Check sheet for the modelled part. Datum: model origin and axes. Units: mm. Face numbers are marked on the shaded views. A direction names the side the tool comes from. Coordinates: 2 decimals unless noted, no trailing zeros. Write each loop counter-clockwise with the first axis right and the second up, starting at its lowest first coordinate (ties: lowest second). Pieces come first, ordered by that corner, then holes. Notation, with made-up numbers: (19.25, -37.75) - (75.25, -37.75) arc R11 ccw to (75.25, -26.75) - close; hole circle Ø10 at (4, 42). An arc over 180 degrees is marked (long way). Answer as CSV lines item,"result". Start each with the question number.
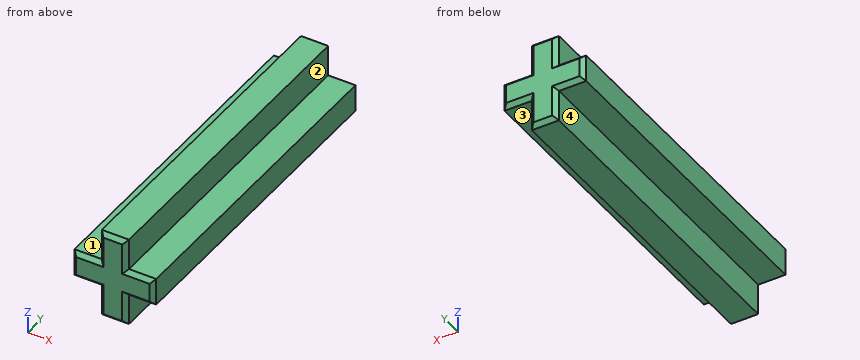
from build123d import *

# Parameters (mm, degrees)
SKETCH1_W           = 1.635
SKETCH1_H           = 1.63
SKETCH1_W_2         = 1.63
SKETCH1_H_2         = 1.87
BOSS_EXTRUDE1_DEPTH = 20
CHAMFER1_SIZE       = 0.25
CHAMFER2_SIZE       = 0.25


with BuildPart() as part:
    # Sketch1 → Boss-Extrude1 (new body)
    with BuildSketch(Plane(origin=(0, 0, 0), x_dir=(1, 0, 0), z_dir=(0, 1, 0))):
        with Locations((-0.8175, 2.685)):
            Rectangle(SKETCH1_W, SKETCH1_H)
        with Locations((0.815, 2.685)):
            Rectangle(SKETCH1_W_2, SKETCH1_H)
        with Locations((0.815, 4.435)):
            Rectangle(SKETCH1_W_2, SKETCH1_H_2)
        with Locations((2.4475, 2.685)):
            Rectangle(SKETCH1_W, SKETCH1_H)
        with Locations((0.815, 0.935)):
            Rectangle(SKETCH1_W_2, SKETCH1_H_2)
    extrude(amount=BOSS_EXTRUDE1_DEPTH)

    # Chamfer1
    chamfer1_edges = [part.edges().sort_by_distance(p)[0] for p in [
        (-0.8175, 20, -1.87),
        (0, 20, -0.935),
        (0.815, 20, 0),
        (1.63, 20, -0.935),
        (2.4475, 20, -1.87),
        (3.265, 20, -2.685),
        (2.4475, 20, -3.5),
        (1.63, 20, -4.435),
        (-1.635, 20, -2.685),
        (0.815, 20, -5.37),
        (0, 20, -4.435),
        (-0.8175, 20, -3.5),
    ]]
    chamfer(chamfer1_edges, length=CHAMFER1_SIZE)

    # Chamfer2
    chamfer2_edges = [part.edges().sort_by_distance(p)[0] for p in [
        (-0.8175, 0, -3.5),
        (0, 0, -4.435),
        (0.815, 0, -5.37),
        (1.63, 0, -4.435),
        (2.4475, 0, -3.5),
        (3.265, 0, -2.685),
        (2.4475, 0, -1.87),
        (1.63, 0, -0.935),
        (0.815, 0, 0),
        (0, 0, -0.935),
        (-0.8175, 0, -1.87),
        (-1.635, 0, -2.685),
    ]]
    chamfer(chamfer2_edges, length=CHAMFER2_SIZE)


solid = part.part
(1) Tool access check on the marked faces 1, 2, 3 and 4. Record the directions out of +Z, -Z, +X, -X, +Y, -Y that give a thin tool (end or side, any length) a straight path to the whole face; none if there is none.
(2) Material ranges on probe 1 along X at (y, z) = (12.5, -1.1); probe 2 along Z at (x, y) = (2.8, 6); probe 3 along Y at (x, z) = (1.4, -0.3), recorded low to high. Write a range as from..to.
(3) Cross-section at A-A on z = -4.4. Record the boundary of the cut face in (x, y).
(4) Go/stop test with flat-tipped pins: P1, Ø0.5, axis at x = -1, y = 9, coming from the -Z side; P2, Ø1.3, axis at x = -1, y = 9.5, coming from the +Z side; P3, Ø0.9, axis at y = 14.5, z = -1, coming from the -X side. Record where each tip stops, or that it passes through.
(5) Cross-section at C-C on x = 1.95. Record the boundary of the cut face in (y, z), plus the area to 3 significant figures.
(6) Cross-section at B-B on y = 12.25. Record the boundary of the cut face in (x, z) (3 decimals), plus the area to 3 significant figures.
Checked values:
1,face 1,"+Z, -X, +Y, -Y"
1,face 2,"+Z, +X, +Y, -Y"
1,face 3,"-Z, +X, +Y, -Y"
1,face 4,"-Z, -X, +Y, -Y"
2,probe 1,"0..1.63"
2,probe 2,"-3.5..-1.87"
2,probe 3,"0.02..19.98"
3,outline,"(0, 0.25) - (0.25, 0) - (1.38, 0) - (1.63, 0.25) - (1.63, 19.75) - (1.38, 20) - (0.25, 20) - (0, 19.75) - close"
4,P1,"z = -3.5"
4,P2,"z = -1.87"
4,P3,"x = 0"
5,outline,"(0, -3.25) - (0.25, -3.5) - (19.75, -3.5) - (20, -3.25) - (20, -2.12) - (19.75, -1.87) - (0.25, -1.87) - (0, -2.12) - close"
5,area,"32.5 mm^2"
6,outline,"(-1.635, -3.5) - (0, -3.5) - (0, -5.37) - (1.63, -5.37) - (1.63, -3.5) - (3.265, -3.5) - (3.265, -1.87) - (1.63, -1.87) - (1.63, 0) - (0, 0) - (0, -1.87) - (-1.635, -1.87) - close"
6,area,"14.1 mm^2"
